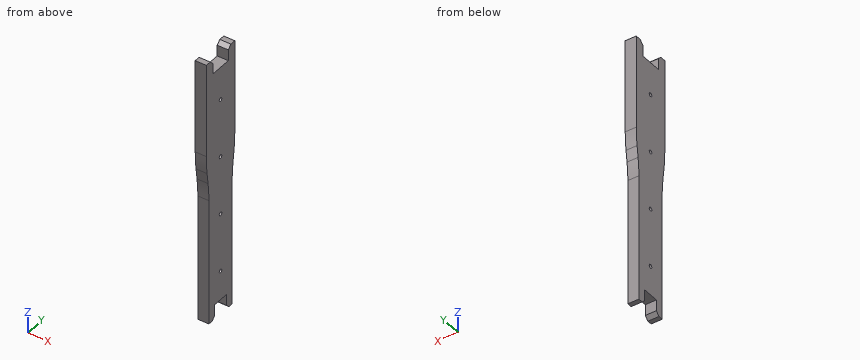
```python
from build123d import *

# Parameters (mm, degrees)
F0_W     = 34.925
F0_H     = 231.775
F1_DEPTH = 9.525
F3_DEPTH = 9.525
F4_R     = 127
F5_W     = 19.05
F5_H     = 12.7
F5_W_2   = 14.2875
F6_DEPTH = 9.525
F7_SIZE  = 3.175
F9_D     = 3.175


# Not quite as in the source:
# - a pattern or mirror of a feature is missing from the dataset's text; its kind, count and spacing are read off the source's solid


with BuildPart() as f1:
    # F0 (on Right) → F1 (new body)
    with BuildSketch(Plane.YZ):
        with Locations((0, 115.8875)):
            Rectangle(F0_W, F0_H)
    extrude(amount=-F1_DEPTH)

    # F2 (on face) → F3 (cut, through all)
    with BuildSketch(Plane.YZ):
        Polygon((14.2875, 117.475), (14.2875, 0), (17.4625, 0), (17.4625, 142.875), align=None)
    f3 = extrude(amount=-F3_DEPTH, mode=Mode.SUBTRACT)

    # F3_copies: F3 across plane
    add(f3.mirror(Plane(origin=(0, 0, 0), x_dir=(0, 0, -1), z_dir=(0, -1, 0))), mode=Mode.SUBTRACT)

    # F4
    f4_edges = [f1.edges().sort_by_distance(p)[0] for p in [
        (-4.7625, 14.2875, 117.475),
        (-4.7625, 17.4625, 142.875),
        (-4.7625, -17.4625, 142.875),
        (-4.7625, -14.2875, 117.475),
    ]]
    fillet(f4_edges, radius=F4_R)

    # F5 (on face) → F6 (cut, through all)
    with BuildSketch(Plane.YZ):
        with Locations((0, 225.425)):
            Rectangle(F5_W, F5_H)
        with Locations((0, 6.35)):
            Rectangle(F5_W_2, F5_H)
    extrude(amount=-F6_DEPTH, mode=Mode.SUBTRACT)

    # F7
    f7_edges = [f1.edges().sort_by_distance(p)[0] for p in [
        (-4.7625, -9.525, 231.775),
        (-4.7625, 9.525, 231.775),
        (-4.7625, -7.14375, 0),
        (-4.7625, 7.14375, 0),
    ]]
    chamfer(f7_edges, length=F7_SIZE)

    # F9 (through all)
    with Locations(Plane.YZ):
        with Locations((0, 139.7), (0, 88.9), (0, 190.5), (0, 38.1)):
            Hole(F9_D / 2)


solid = f1.part
```
Can you work these out from the model? Positions are in its coordinate system, mm. Give positions to 0.01 mm unless a question says otherwise; leave off trailing zeros. Order: outer loops, then holes, each group sorted by start corner. A loop starts at its lowest first (then second) coordinate and runs counter-clockwise, first axis right, second up. Notation, with made-up numbers: (52, 67) - (111, 67) arc R27 ccw to (111, 86) - close; hole circle Ø1 at (23, 58.5). An arc over 180 degrees is marked (long way). Use a Markdown table: item, result. Add a question column.
Q1. If we section it at A-A on x = -3.75: Write out the boundary of the cut face in (y, z) (1 decimal).
Q2. If we section it at B-B on y = 5: Write out the boundary of the cut face in (x, z) (3 decimals), plus the area to 3 significant figures.
Q3. I'm going to push flat-ended pins straight in: pin 1 (3 mm diameter, centred on x = -5, z = 34, fed in from -Y); pin 2 (5 mm diameter, centred on x = -6.5, z = 44.5, fed in from +Y). Where does each tip first touch, or does it pass through?
Q4. Please list where these lines run through material, in increasing order: line 1 along Z through (x, y) = (-5, 0) (1 decimal); line 2 along Y through (x, z) = (-2.5, 88.9); line 3 along Y through (x, z) = (-5, 74.5).
Q5. If we section it at C-C on z = 58: Write out the boundary of the cut face in (x, y) (1 decimal), plus the area to 3 significant figures.
Answers follow:
| question | item | result |
|---|---|---|
| 1 | outline | (-17.5, 150.8) arc R127 ccw to (-16.5, 135) - (-15.3, 125.3) arc R127 cw to (-14.3, 109.6) - (-14.3, 0) - (-10.3, 0) - (-7.1, 3.2) - (-7.1, 12.7) - (7.1, 12.7) - (7.1, 3.2) - (10.3, 0) - (14.3, 0) - (14.3, 109.6) arc R127 cw to (15.3, 125.3) - (16.5, 135) arc R127 ccw to (17.5, 150.8) - (17.5, 231.8) - (12.7, 231.8) - (9.5, 228.6) - (9.5, 219.1) - (-9.5, 219.1) - (-9.5, 228.6) - (-12.7, 231.8) - (-17.5, 231.8) - close; hole circle Ø3.2 at (0, 38.1); hole circle Ø3.2 at (0, 88.9); hole circle Ø3.2 at (0, 139.7); hole circle Ø3.2 at (0, 190.5) |
| 2 | outline | (-9.525, 12.7) - (0, 12.7) - (0, 219.075) - (-9.525, 219.075) - close |
| 2 | area | 1,970 mm^2 |
| 3 | pin 1 | stops at y = -14.29 |
| 3 | pin 2 | stops at y = 14.29 |
| 4 | line 1 | z = 12.7 to 36.5, 39.7 to 87.3, 90.5 to 138.1, 141.3 to 188.9, 192.1 to 219.1 |
| 4 | line 2 | y = -14.29 to -1.59, 1.59 to 14.29 |
| 4 | line 3 | y = -14.29 to 14.29 |
| 5 | outline | (-9.5, -14.3) - (0, -14.3) - (0, 14.3) - (-9.5, 14.3) - close |
| 5 | area | 272 mm^2 |
